Check sheet for the modelled part. Datum: model origin and axes. Units: mm. Round coordinates to 2 decimals unless told otherwise and drop trailing zeros. Order: outer loops, then holes, each group sorted by start corner. A loop starts at its lowest first (then second) coordinate and runs counter-clockwise, first axis right, second up. Notation, with made-up numbers: (26.25, 12) -> (33.25, 12) arc R20 cw to (33.25, 23) -> close; hole circle Ø3 at (9.5, 16). An arc over 180 degrees is marked (long way). Use CSV: the item, a comma, the result in double quotes.
```python
from build123d import *

# Parameters (mm, degrees)
F0_R     = 12.7
F1_DEPTH = 279.4
F2_R     = 184.15
F2_R_2   = 12.7
F3_DEPTH = 76.2
F4_R     = 184.15
F4_R_2   = 12.7
F5_DEPTH = 71.12


with BuildPart() as f1:
    # F0 (on Right) → F1 (new body, symmetric)
    with BuildSketch(Plane.YZ):
        Circle(F0_R)
    extrude(amount=F1_DEPTH, both=True)

    # F2 (on face) → F3 (join)
    with BuildSketch(Plane.YZ.offset(279.4)):
        Circle(F2_R)
        Circle(F2_R_2, mode=Mode.SUBTRACT)
    extrude(amount=-F3_DEPTH)

    # F4 (on face) → F5 (join)
    with BuildSketch(Plane(origin=(-279.4, 0, 0), x_dir=(0, -1, 0), z_dir=(-1, 0, 0))):
        Circle(F4_R)
        Circle(F4_R_2, mode=Mode.SUBTRACT)
    extrude(amount=-F5_DEPTH)


solid = f1.part
```
Q1. Sectioned sample at A-A, the plane y = -64.5. Enter the section's corners in (x, z).
Result sheet:
outline,"(-279.4, -172.48) -> (-208.28, -172.48) -> (-208.28, 172.48) -> (-279.4, 172.48) -> close; (203.2, -172.48) -> (279.4, -172.48) -> (279.4, 172.48) -> (203.2, 172.48) -> close"
Q2. Scan lines: L1, parallel to X at y = 99, z = 74.5; L2, parallel to Y at x = 210, z = -96.5; L3, parallel to Y at x = -249, z = 97. Record each from-to range of solid material in increasing order.
Result sheet:
L1,"x = -279.4 to -208.28, 203.2 to 279.4"
L2,"y = -156.84 to 156.84"
L3,"y = -156.53 to 156.53"
Q3. Sectioned sample at B-B, the plane z = -107. Enter the section's corners in (x, y).
Result sheet:
outline,"(-279.4, -149.87) -> (-208.28, -149.87) -> (-208.28, 149.87) -> (-279.4, 149.87) -> close; (203.2, -149.87) -> (279.4, -149.87) -> (279.4, 149.87) -> (203.2, 149.87) -> close"
Q4. Sectioned sample at C-C, the plane y = 0. Enter the section's corners in (x, z), then the cut area to 3 significant figures.
Result sheet:
outline,"(-279.4, -184.15) -> (-208.28, -184.15) -> (-208.28, -12.7) -> (203.2, -12.7) -> (203.2, -184.15) -> (279.4, -184.15) -> (279.4, 184.15) -> (203.2, 184.15) -> (203.2, 12.7) -> (-208.28, 12.7) -> (-208.28, 184.15) -> (-279.4, 184.15) -> close"
area,"64,700 mm^2"
Q5. Mould release check, pull along X, two halves, no side actions. Record for faces 1 (the face through (241.8, -146.1, -112.1)), 2 (the face through (0.34, -2.75, -12.4)), 3 (the face through (279.4, -3, 3)): pulls with the +X half, pulls with the -X half, needs draft (parallel to the pull), parting line crosses it, or undercut.
Result sheet:
face 1,"needs draft"
face 2,"undercut"
face 3,"pulls with the +X half"
Q6. Go/stop test with a flat-tipped pin: pin 1 (6 mm diameter, centred on x = 102.5, z = 2.5, fed in from -Y). Record where the tip stops, or that it passes through.
Result sheet:
pin 1,"stops at y = -12.7"
